Here's how the part is built. I have some questions about the finished solid (model axes, mm). A direction names the side the tool comes from. Coordinates: 2 decimals unless noted, no trailing zeros. Loops run counter-clockwise (first coordinate to the right, second up) from the corner with the lowest first, then second, coordinate; pieces in that order, holes last. Notation, with made-up numbers: M -18.75,-4 L 21.25,-4 A29 ccw 21.25,29 Z; hole C 38.5,57 d11. An arc over 180 degrees is marked long. Use CSV: the item, a comma, the result in double quotes. Start each with the question number.
Q1. For pin 1 Ø1 at (y, z) = (14, 2.5) entering from -X; pin 2 Ø2.5 at (x, y) = (0, -30) entering from -Z; pin 3 Ø6.5 at (x, y) = (0, -30) entering from +Z; pin 4 Ø2 at (y, z) = (6.5, 1.5) entering from -X, each with a flat end and sliding along its axis, tell me the tip position at first contact or that it passes through.
Q2. If we mould it in two halves opening along X, with no side actions, what happens to faces 1 (the flat face through (16, -16, 0)), 2 (the cylindrical face through (-4.88, 37.18, 2.76)), 3 (the cylindrical face through (0, -29, 1))? For each: +X half, -X half, draft (parallel to the pull), parting line (faces both ways), or undercut.
Q3. If we section it at B-B (x = 30): Please give me the cut outline in (y, z).
Q4. If we section it at A-A (y = 0): Please give me the cut outline in (x, z).
Q5. If we section it at C-C (z = 3.9): State how many separate pieces and enclosed holes the cut face has, and give its area (3 significant figures).
Q6. Please list where these lines run through material, in increasing order: probe 1 along Y at (x, z) = (0, 4.7); probe 2 along X at (y, z) = (24.5, 3.3); probe 3 along X at (y, z) = (-18, 3.25). Write a range as [from, to].
Q7. Which directions (+Z, -Z, +X, -X, +Y, -Y) give clear straight access to the entire face, cutting with the end or side of a thin tool? Please do faces 4 (the cylindrical face through (23, -22, 1)), 5 (the cylindrical face through (-0.521, -26.034, 4.079)).
from build123d import *

# Parameters (mm, degrees)
SKETCH_1_R      = 37.5
SKETCH_1_R_2    = 20
SKETCH_1_R_3    = 1
EXTRUDE_1_DEPTH = 2
SKETCH_2_R      = 37.5
SKETCH_2_R_2    = 17.5
SKETCH_2_R_3    = 1
EXTRUDE_2_DEPTH = 0.6
SKETCH_3_R      = 37.5
SKETCH_3_R_2    = 17.5
SKETCH_3_R_3    = 4
EXTRUDE_3_DEPTH = 3


with BuildPart() as part:
    # Эскиз1 → Бобышка-Вытянуть1 (new body)
    with BuildSketch(Plane.XY):
        Circle(SKETCH_1_R)
        Circle(SKETCH_1_R_2, mode=Mode.SUBTRACT)
        with Locations((0, 30)):
            Circle(SKETCH_1_R_3, mode=Mode.SUBTRACT)
        with Locations((0, -30)):
            Circle(SKETCH_1_R_3, mode=Mode.SUBTRACT)
        with Locations((30, 0)):
            Circle(SKETCH_1_R_3, mode=Mode.SUBTRACT)
        with Locations((-30, 0)):
            Circle(SKETCH_1_R_3, mode=Mode.SUBTRACT)
        with Locations((23, 21)):
            Circle(SKETCH_1_R_3, mode=Mode.SUBTRACT)
        with Locations((-23, 21)):
            Circle(SKETCH_1_R_3, mode=Mode.SUBTRACT)
        with Locations((-23, -21)):
            Circle(SKETCH_1_R_3, mode=Mode.SUBTRACT)
        with Locations((23, -21)):
            Circle(SKETCH_1_R_3, mode=Mode.SUBTRACT)
    extrude(amount=EXTRUDE_1_DEPTH)

    # Эскиз2 → Бобышка-Вытянуть2 (add)
    with BuildSketch(Plane.XY.offset(2)):
        Circle(SKETCH_2_R)
        Circle(SKETCH_2_R_2, mode=Mode.SUBTRACT)
        with Locations((0, 30)):
            Circle(SKETCH_2_R_3, mode=Mode.SUBTRACT)
        with Locations((0, -30)):
            Circle(SKETCH_2_R_3, mode=Mode.SUBTRACT)
        with Locations((-30, 0)):
            Circle(SKETCH_2_R_3, mode=Mode.SUBTRACT)
        with Locations((30, 0)):
            Circle(SKETCH_2_R_3, mode=Mode.SUBTRACT)
        with Locations((-23, 21)):
            Circle(SKETCH_2_R_3, mode=Mode.SUBTRACT)
        with Locations((23, 21)):
            Circle(SKETCH_2_R_3, mode=Mode.SUBTRACT)
        with Locations((23, -21)):
            Circle(SKETCH_2_R_3, mode=Mode.SUBTRACT)
        with Locations((-23, -21)):
            Circle(SKETCH_2_R_3, mode=Mode.SUBTRACT)
    extrude(amount=EXTRUDE_2_DEPTH)

    # Эскиз3 → Бобышка-Вытянуть3 (add)
    with BuildSketch(Plane.XY.offset(2.6)):
        Circle(SKETCH_3_R)
        Circle(SKETCH_3_R_2, mode=Mode.SUBTRACT)
        with Locations((0, 30)):
            Circle(SKETCH_3_R_3, mode=Mode.SUBTRACT)
        with Locations((0, -30)):
            Circle(SKETCH_3_R_3, mode=Mode.SUBTRACT)
        with Locations((30, 0)):
            Circle(SKETCH_3_R_3, mode=Mode.SUBTRACT)
        with Locations((-30, 0)):
            Circle(SKETCH_3_R_3, mode=Mode.SUBTRACT)
        with Locations((23, 21)):
            Circle(SKETCH_3_R_3, mode=Mode.SUBTRACT)
        with Locations((-23, 21)):
            Circle(SKETCH_3_R_3, mode=Mode.SUBTRACT)
        with Locations((-23, -21)):
            Circle(SKETCH_3_R_3, mode=Mode.SUBTRACT)
        with Locations((23, -21)):
            Circle(SKETCH_3_R_3, mode=Mode.SUBTRACT)
    extrude(amount=EXTRUDE_3_DEPTH)


solid = part.part
Results below:
1,pin 1,"x = -34.99"
1,pin 2,"z = 0"
1,pin 3,"z = 2.6"
1,pin 4,"x = -37.09"
2,face 1,"draft"
2,face 2,"parting line"
2,face 3,"undercut"
3,outline,"M -22.5,0 L -1,0 L -1,2.6 L -4,2.6 L -4,5.6 L -22.5,5.6 Z; M 1,0 L 22.5,0 L 22.5,5.6 L 4,5.6 L 4,2.6 L 1,2.6 Z"
4,outline,"M -37.5,0 L -31,0 L -31,2.6 L -34,2.6 L -34,5.6 L -37.5,5.6 Z; M -29,0 L -20,0 L -20,2 L -17.5,2 L -17.5,5.6 L -26,5.6 L -26,2.6 L -29,2.6 Z; M 17.5,2 L 20,2 L 20,0 L 29,0 L 29,2.6 L 26,2.6 L 26,5.6 L 17.5,5.6 Z; M 31,0 L 37.5,0 L 37.5,5.6 L 34,5.6 L 34,2.6 L 31,2.6 Z"
5,separate pieces,"1"
5,enclosed holes,"9"
5,area,"3,050 mm^2"
6,probe 1,"[-37.5, -34], [-26, -17.5], [17.5, 26], [34, 37.5]"
6,probe 2,"[-28.39, -24.94], [-21.06, 21.06], [24.94, 28.39]"
6,probe 3,"[-32.9, -25.65], [-20.35, 20.35], [25.65, 32.9]"
7,face 4,"+Z, -Z"
7,face 5,"+Z"
